```python
from build123d import *

# Parameters (mm, degrees)
F0_W     = 203.2
F0_H     = 152.4
F1_DEPTH = 203.2
F2_W     = 152.4
F2_H     = 101.6
F3_DEPTH = 203.201
F4_R     = 5.08
F5_W     = 44.45
F5_H     = 25.4
F6_DEPTH = 203.2


with BuildPart() as f1:
    # F0 (on Top) → F1 (new body)
    with BuildSketch(Plane.XY):
        Rectangle(F0_W, F0_H)
    extrude(amount=F1_DEPTH)

    # F2 (on face) → F3 (cut, through all)
    with BuildSketch(Plane.XY.offset(203.2)):
        Rectangle(F2_W, F2_H)
    extrude(amount=-F3_DEPTH, mode=Mode.SUBTRACT)

    # F4
    f4_edges = [f1.edges().sort_by_distance(p)[0] for p in [
        (-76.2, 0, 203.2),
        (-76.2, -50.8, 101.6),
        (-76.2, 0, 0),
        (-76.2, 50.8, 101.6),
        (0, -50.8, 203.2),
        (76.2, -50.8, 101.6),
        (0, -50.8, 0),
        (76.2, 0, 203.2),
        (76.2, 50.8, 101.6),
        (76.2, 0, 0),
        (0, 50.8, 203.2),
        (0, 50.8, 0),
    ]]
    fillet(f4_edges, radius=F4_R)

    # F5 (on face) → F6 (cut)
    with BuildSketch(Plane.YZ.offset(101.6)):
        with Locations((0, 190.5)):
            Rectangle(F5_W, F5_H)
    extrude(amount=-F6_DEPTH, mode=Mode.SUBTRACT)


solid = f1.part
```
Verification items for the finished model (mm, model axes). A direction names the side the tool comes from. Coordinates: 2 decimals unless noted, no trailing zeros. Order: outer loops, then holes, each group sorted by start corner. A loop starts at its lowest first (then second) coordinate and runs counter-clockwise, first axis right, second up. Notation, with made-up numbers: (61.5, 37.5) - (85.5, 37.5) arc R5 ccw to (85.5, 41.5) - close; hole circle Ø10 at (3, -7). An arc over 180 degrees is marked (long way). Return JSON: item names as keys, results as strings.
(1) Mould release check, pull along Y, two halves, no side actions. Record for faces 1 (the cylindrical face through (-78, 34, 202)), 2 (the flat face through (-101.6, -1, 100)): pulls with the +Y half, pulls with the -Y half, needs draft (parallel to the pull), parting line crosses it, or undercut.
Filled sheet:
{"face 1": "undercut", "face 2": "needs draft"}
(2) Access from +Z, -Z, +X, -X, +Y, -Y to the whole of each face (thin tool, end or side, straight path). Record for faces 3 (the cylindrical face through (0.996, -52.328, 201.751)), 4 (the cylindrical face through (-77.728, 0.64, 1.449)), 5 (the flat face through (89, -22.225, 190)), 6 (the flat face through (76.2, -1, 103)).
Filled sheet:
{"face 3": "+Z", "face 4": "-Z", "face 5": "+Z, +X, -X", "face 6": "+Z, -Z"}
(3) Go/stop test with a flat-tipped pin: pin 1 (12.5 mm diameter, centred on x = -88, y = 5.5, fed in from +Z). Record where the tip stops, or that it passes through.
Filled sheet:
{"pin 1": "stops at z = 177.8"}
(4) Section check B-B, the plane x = -24. Record the cut outline in (y, z), and give its area (3 significant figures).
Filled sheet:
{"outline": "(-76.2, 0) - (-55.88, 0) arc R5.08 ccw to (-50.8, 5.08) - (-50.8, 198.12) arc R5.08 ccw to (-55.88, 203.2) - (-76.2, 203.2) - close; (50.8, 5.08) arc R5.08 ccw to (55.88, 0) - (76.2, 0) - (76.2, 203.2) - (55.88, 203.2) arc R5.08 ccw to (50.8, 198.12) - close", "area": "10,300 mm^2"}
(5) Thickness scan on line 1 along Y through (x, z) = (-40.5, 187); line 2 along X through (y, z) = (38.5, 115); line 3 along X through (y, z) = (-49, 50). Record the ranges inside material, lowest first.
Filled sheet:
{"line 1": "y = -76.2 to -50.8, 50.8 to 76.2", "line 2": "x = -101.6 to -76.2, 76.2 to 101.6", "line 3": "x = -101.6 to -75, 75 to 101.6"}
(6) Section check C-C, the plane z = 128. Record the cut outline in (x, y).
Filled sheet:
{"outline": "(-101.6, -76.2) - (101.6, -76.2) - (101.6, 76.2) - (-101.6, 76.2) - close; hole (-76.2, -45.72) arc R5.08 ccw to (-71.12, -50.8) - (71.12, -50.8) arc R5.08 ccw to (76.2, -45.72) - (76.2, 45.72) arc R5.08 ccw to (71.12, 50.8) - (-71.12, 50.8) arc R5.08 ccw to (-76.2, 45.72) - close"}
(7) Section check A-A, the plane y = -27.5. Record the cut outline in (x, z).
Filled sheet:
{"outline": "(-101.6, 0) - (-81.28, 0) arc R5.08 ccw to (-76.2, 5.08) - (-76.2, 198.12) arc R5.08 ccw to (-81.28, 203.2) - (-101.6, 203.2) - close; (76.2, 5.08) arc R5.08 ccw to (81.28, 0) - (101.6, 0) - (101.6, 203.2) - (81.28, 203.2) arc R5.08 ccw to (76.2, 198.12) - close"}
(8) Section check D-D, the plane x = 86. Record the cut outline in (y, z) (3 decimals).
Filled sheet:
{"outline": "(-76.2, 0) - (76.2, 0) - (76.2, 203.2) - (22.225, 203.2) - (22.225, 177.8) - (-22.225, 177.8) - (-22.225, 203.2) - (-76.2, 203.2) - close"}
